Build history of the part. All positions in model axes, mm. A direction names the side the tool comes from. Give positions to 0.01 mm unless a question says otherwise; leave off trailing zeros. Order: outer loops, then holes, each group sorted by start corner. A loop starts at its lowest first (then second) coordinate and runs counter-clockwise, first axis right, second up. Notation, with made-up numbers: (72.5, -17.75) - (92.5, -17.75) arc R14 ccw to (92.5, 5.25) - close; hole circle Ø2 at (-29, 25). An arc over 180 degrees is marked (long way). Answer in a Markdown table with one row per item.
```python
from build123d import *

# Parameters (mm, degrees)
SKETCH_1_R          = 8
EXTRUDE_1_DEPTH     = 6
SKETCH_2_R          = 1.5
SKETCH_2_W          = 14
SKETCH_2_H          = 25
SKETCH_2_H_2        = 30
SKETCH_2_H_3        = 35
SKETCH_2_H_4        = 40
SKETCH_2_H_5        = 18
CUT_EXTRUDE_1_DEPTH = 248.913795502
FILLET_1_R          = 3


with BuildPart() as part:
    # 草图1 → 凸台-拉伸1 (new body)
    with BuildSketch(Plane.XY):
        with BuildLine():
            Line((-13, 0), (-13, 210))
            ThreePointArc((-13, 210), (-11.543396381, 215.979130372), (-7.5, 220.618380291))
            Line((-7.5, 220.618380291), (-7.5, 240))
            ThreePointArc((-7.5, 240), (0, 247.5), (7.5, 240))
            Line((7.5, 240), (7.5, 220.618380291))
            ThreePointArc((7.5, 220.618380291), (11.543396381, 215.979130372), (13, 210))
            Line((13, 210), (13, 0))
            ThreePointArc((13, 0), (0, -13), (-13, 0))
        make_face()
        Circle(SKETCH_1_R, mode=Mode.SUBTRACT)
        with Locations((0, 210)):
            Circle(SKETCH_1_R, mode=Mode.SUBTRACT)
    extrude(amount=EXTRUDE_1_DEPTH)

    # 草图2 → 切除-拉伸1 (cut, through all)
    with BuildSketch(Plane.XY.offset(6)):
        with Locations((0, 233)):
            Circle(SKETCH_2_R)
        with Locations((0, 225)):
            Circle(SKETCH_2_R)
        with Locations((0, 162.5)):
            Rectangle(SKETCH_2_W, SKETCH_2_H)
        with Locations((0, 125)):
            Rectangle(SKETCH_2_W, SKETCH_2_H_2)
        with Locations((0, 82.5)):
            Rectangle(SKETCH_2_W, SKETCH_2_H_3)
        with Locations((0, 35)):
            Rectangle(SKETCH_2_W, SKETCH_2_H_4)
        with Locations((0, 189)):
            Rectangle(SKETCH_2_W, SKETCH_2_H_5)
    extrude(amount=-CUT_EXTRUDE_1_DEPTH, mode=Mode.SUBTRACT)

    # 圆角1
    fillet_1_edges = [part.edges().sort_by_distance(p)[0] for p in [
        (7, 55, 3),
        (7, 15, 3),
        (-7, 15, 3),
        (-7, 55, 3),
        (7, 100, 3),
        (7, 65, 3),
        (-7, 65, 3),
        (-7, 100, 3),
        (7, 140, 3),
        (7, 110, 3),
        (-7, 110, 3),
        (-7, 140, 3),
        (7, 198, 3),
        (7, 180, 3),
        (-7, 180, 3),
        (-7, 198, 3),
        (7, 175, 3),
        (7, 150, 3),
        (-7, 150, 3),
        (-7, 175, 3),
    ]]
    fillet(fillet_1_edges, radius=FILLET_1_R)


solid = part.part
```
1. Probe line 1 (X direction, y = 233, z = 3.55); line 2 (X direction, y = 71, z = 4.25); line 3 (X direction, y = 230, z = 4.75). List the from-to ranges inside material, lowest first.
Check result:
| item | result |
|---|---|
| line 1 | x = -7.5 to -1.5, 1.5 to 7.5 |
| line 2 | x = -13 to -7, 7 to 13 |
| line 3 | x = -7.5 to 7.5 |
2. Cut at C-C on x = 10.25. Write the cut outline in (y, z), and give its area (3 significant figures).
Check result:
| item | result |
|---|---|
| outline | (-8, 0) - (218, 0) - (218, 6) - (-8, 6) - close |
| area | 1,360 mm² |
3. Two-plate mould, pull along Y, no slides. Class faces 1 (the face through (9, 119, 6)), 2 (the face through (7, 162, 3)), 3 (the face through (11.5, 216.06, 2.96)): +Y half, -Y half, draft (parallel to the pull), parting line (faces both ways), or undercut.
Check result:
| item | result |
|---|---|
| face 1 | draft |
| face 2 | undercut |
| face 3 | +Y half |
4. Cut at B-B on z = 3.4. Count the separate pieces of the cut face and the enclosed holes in it, and give its area (3 significant figures).
Check result:
| item | result |
|---|---|
| separate pieces | 1 |
| enclosed holes | 9 |
| area | 3,900 mm² |
5. Which spindle directions (+Z, -Z, +X, -X, +Y, -Y) get a long thin tool onto all of the face, cutting with end or side? Do faces 4 (the face through (7.5, 230, 3)), 5 (the face through (-7, 82, 3)), 6 (the face through (-13, 104, 3)). Say none if no direction does.
Check result:
| item | result |
|---|---|
| face 4 | +Z, -Z, +X, +Y |
| face 5 | +Z, -Z |
| face 6 | +Z, -Z, -X, +Y, -Y |
6. Cut at A-A on y = 117. Write the cut outline in (x, z), and give its area (3 significant figures).
Check result:
| item | result |
|---|---|
| outline | (-13, 0) - (-7, 0) - (-7, 6) - (-13, 6) - close; (7, 0) - (13, 0) - (13, 6) - (7, 6) - close |
| area | 72.0 mm² |
7. Drop flat-ended pins along their axis: P1, Ø3, axis at y = 231.5, z = 2, coming from the +X side; P2, Ø2, axis at x = 3, y = 174.5, coming from the +Z side; P3, Ø2, axis at x = -2, y = 52.5, coming from the -Z side; P4, Ø1, axis at x = 10, z = 1.5, coming from the +Y side. Give the stop position or say it passes through.
Check result:
| item | result |
|---|---|
| P1 | stops at x = 7.5 |
| P2 | stops at z = 6 |
| P3 | passes through |
| P4 | stops at y = 218.87 |
